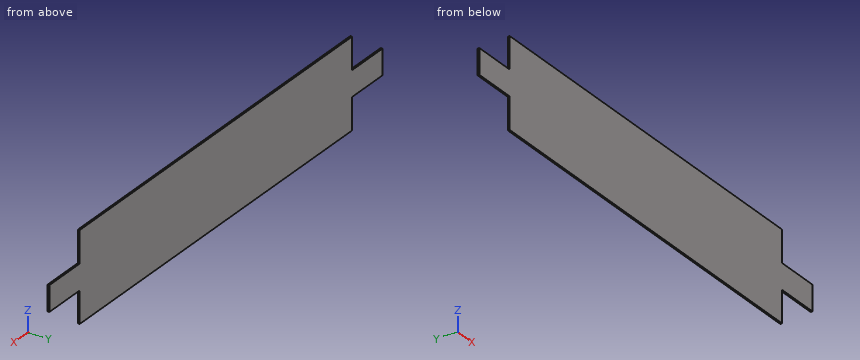
from build123d import *

# Parameters (mm, degrees)
F0_W     = 448
F0_H     = 14
F0_H_2   = 21
F0_H_3   = 28
F0_W_2   = 50
F1_DEPTH = 2


with BuildPart() as f1:
    # F0 (on Front) → F1 (new body)
    with BuildSketch(Plane.XZ):
        with Locations((0, 42)):
            Rectangle(F0_W, F0_H)
        with Locations((0, 24.5)):
            Rectangle(F0_W, F0_H_2)
        Rectangle(F0_W, F0_H_3)
        with Locations((-249, 0)):
            Rectangle(F0_W_2, F0_H_3)
        with Locations((0, -21)):
            Rectangle(F0_W, F0_H)
        with Locations((0, -38.5)):
            Rectangle(F0_W, F0_H_2)
        with Locations((249, 0)):
            Rectangle(F0_W_2, F0_H_3)
    extrude(amount=F1_DEPTH)


solid = f1.part
Read the model definition and answer for the solid it produces. Units are mm, in the model's axes. Round coordinates to 2 decimals unless told otherwise and drop trailing zeros. Write each loop counter-clockwise with the first axis right and the second up, starting at its lowest first coordinate (ties: lowest second). Pieces come first, ordered by that corner, then holes.
1. The part is cut by section B-B, the plane z = 27.5. Determine the outline of the cut face in (x, y).
2. The part is cut by section A-A, the plane y = -1.5. Determine the outline of the cut face in (x, z).
3. Given pin 1 Ø0.6 at (y, z) = (-0.5, -34.5) entering from +X; pin 2 Ø1 at (y, z) = (-1, 34.5) entering from -X, each flat-ended and moving along its own axis, determine where each tip first touches the part or whether it passes through.
4. A straight line is drawn through the part: L1, parallel to X at y = -1.4, z = -35.5. Find the intervals that lie inside material, in ascending order.
Values:
1. outline: (-224, -2) - (224, -2) - (224, 0) - (-224, 0) - close
2. outline: (-274, -14) - (-224, -14) - (-224, -49) - (224, -49) - (224, -14) - (274, -14) - (274, 14) - (224, 14) - (224, 49) - (-224, 49) - (-224, 14) - (-274, 14) - close
3. pin 1: stops at x = 224
3. pin 2: stops at x = -224
4. L1: x = -224 to 224
